Autodesk Inventor part; units mm, degrees
ref_plane "Work Plane1" through (-5, 47, 0) normal (0.7071, 0.7071, 0) x (0, 0, -1)
ref_plane "CentrePlane" through (8, 0, 0) normal (1, 0, 0) x (0, 0, -1)
ref_plane "YZ Plane" through (0, 0, 0) normal (1, 0, 0) x (0, 1, 0)
sketch "Sketch1" plane through (0, 0, 0) normal (0, 0, 1) x (1, 0, 0)
  line L0 (0, 0) -> (16, 0) construction
  line L1 (16, 0) -> (16, 8) construction
  line L2 (0, 8) -> (0, 0) construction
  line L3 (5.5, 10.5) -> (0, 10.5) construction
  line L4 (0, 10.5) -> (0, 8) construction
  line L5 (13.5, 10.5) -> (16, 10.5) construction
  line L6 (16, 10.5) -> (16, 8) construction
  line L7 (6.5, 37) -> (12.5, 37) construction
  line L8 (12.5, 37) -> (12.5, 8) construction
  line L9 (12.5, 8) -> (6.5, 8) construction
  line L10 (6.5, 8) -> (6.5, 37) construction
  line L11 (0.5, 34.5) -> (15.5, 34.5) construction
  line L12 (15.5, 34.5) -> (15.5, 10.5) construction
  line L13 (15.5, 10.5) -> (0.5, 10.5) construction
  line L14 (0.5, 10.5) -> (0.5, 34.5) construction
  line L15 (-2, 0) -> (-2, 39)
  line L16 (-2, 39) -> (18, 39)
  line L17 (8, -29.8106) -> (8, -55.1885) construction
  line L18 (-5, 47) -> (-5, 0)
  line L19 (-2, 0) -> (-5, 0)
  line L20 (-5, 47) -> (10, 47)
  line L21 (21, 47) -> (21, 0)
  line L22 (18, 0) -> (21, 0)
  line L23 (21, 47) -> (10, 47)
  line L24 (18, 0) -> (18, 39)
  line L25 (16.05, 25.6) -> (16.05, 19.4) construction
  line L26 (-0.05, 19.4) -> (-0.05, 25.6) construction
  line L27 (-0.05, 25.6) -> (0.5, 25.6) construction
  line L28 (16.05, 25.6) -> (15.5, 25.6) construction
  line L29 (16.05, 19.4) -> (15.5, 19.4) construction
  line L30 (-0.05, 19.4) -> (0.5, 19.4) construction
  line L31 (16.05, 22.5) -> (-0.05, 22.5) construction
  line L32 (0, 8) -> (16, 8) construction
  line L33 (5.5, 10.5) -> (5.5, 8) construction
  line L34 (13.5, 10.5) -> (13.5, 8) construction
  line L35 (5.5, 8) -> (13.5, 8) construction
  point P0 (6.5, 22.5)
  point P1 (0.5, 22.5)
  point P2 (9.5, 8)
  point P3 (8, 0)
  point P4 (8, 39)
  point P5 (8, -42.4996)
  point P6 (9.5, 8)
  point P7 (8, 22.5)
  dimension "d1" = 16
  dimension "d7" = 6
  dimension "d9" = 6
  dimension "d10" = 3
  dimension "d11" = 29
  dimension "d12" = 24
  dimension "d20" = 2
  dimension "thickness" = 3
  dimension "d23" = 8
  dimension "d31" = 22.5
  dimension "d40" = 24.5
  dimension "d41" = 39
  dimension "d60" = 6.2
  dimension "d62" = 16.1
  dimension "d63" = 8
  dimension "d64" = 8
  dimension "d65" = 1
  dimension "d66" = 2.5
  dimension "d97" = 2
extrude "LENGTH" add sketch "Sketch1" against normal blind 73.5
sketch "Sketch2" plane through (-5, 0, 0) normal (-1, 0, 0) x (0, 0, 1)
  circle A0 centre (-12, 22.5) radius 3
  circle A1 centre (-61.5, 22.5) radius 3
  line L0 (-73.5, 0) -> (-73.5, 47) construction
  line L1 (0, 47) -> (0, 0) construction
  dimension "d26" = 6
  dimension "d28" = 6
  dimension "d29" = 12
  dimension "d30" = 12
  dimension "d32" = 22.5
extrude "Extrusion2" cut sketch "Sketch2" against normal through all
ref_plane "Work Plane1" through (-5, 47, 0) normal (0.7071, 0.7071, 0) x (0, 0, -1)
ref_plane "CentrePlane" through (8, 0, 0) normal (1, 0, 0) x (0, 0, -1)
sketch "Measurements" plane through (-5, 0, 0) normal (-1, 0, 0) x (0, 0, 1)
  line L0 (-18.9044, 8) -> (-18.9044, 0) construction
  line L1 (0, 0) -> (0, 8) construction
  spline S0 degree 3 poles (-18.9044, 0) (-18.8729, 0.004) (-18.7747, 0.0145) (-18.6089, 0.0198) (-18.4076, 0.0173) (-18.2077, -0.0064) (-18.0095, -0.0413) (-17.7511, -0.1137) (-17.4304, -0.2111) (-17.1073, -0.2999) (-16.8501, -0.3765) (-16.6638, -0.4528) (-16.4821, -0.5394) (-16.3106, -0.6447) (-16.1439, -0.7575) (-15.9893, -0.8866) (-15.8435, -1.0251) (-15.7068, -1.1728) (-15.5834, -1.3319) (-15.4695, -1.4977) (-15.3662, -1.6705) (-15.2464, -1.9105) (-15.1208, -2.2219) (-15.0142, -2.6104) (-14.9462, -3.0072) (-14.9104, -3.408) (-14.9034, -3.8104) (-14.9258, -4.2123) (-14.9692, -4.6123) (-15.0344, -5.0094) (-15.0913, -5.2714) (-15.1198, -5.4024) knots -0.847201 -0.847201 -0.847201 -0.847201 -0.83705 -0.815587 -0.794126 -0.772659 -0.751201 -0.729734 -0.686802 -0.64387 -0.622403 -0.600945 -0.579478 -0.558017 -0.536554 -0.515088 -0.49363 -0.472163 -0.450698 -0.429238 -0.407769 -0.386302 -0.343394 -0.300476 -0.257562 -0.214646 -0.17172 -0.12879 -0.085861 -0.04293 0 0 0 0 construction
  spline S1 degree 3 poles (-4.5152, -5.4024) (-4.5336, -5.2605) (-4.5704, -4.9766) (-4.6037, -4.5484) (-4.6135, -4.119) (-4.6009, -3.6896) (-4.557, -3.2623) (-4.4825, -2.8392) (-4.3742, -2.4233) (-4.2256, -2.0199) (-4.0637, -1.7) (-3.9145, -1.4557) (-3.7891, -1.2813) (-3.6528, -1.1153) (-3.5072, -0.9573) (-3.3484, -0.8126) (-3.1807, -0.6785) (-3.0046, -0.5552) (-2.8172, -0.4504) (-2.6251, -0.3539) (-2.424, -0.2783) (-2.219, -0.214) (-1.9385, -0.1559) (-1.5868, -0.0908) (-1.2369, -0.0163) (-0.9555, 0.0373) (-0.7415, 0.0564) (-0.5268, 0.0635) (-0.3125, 0.0479) (-0.1366, 0.0272) (-0.0331, 0.0071) (0, 0) knots -1.373604 -1.373604 -1.373604 -1.373604 -1.330674 -1.287743 -1.244814 -1.201884 -1.158958 -1.116042 -1.073128 -1.03021 -0.987302 -0.965835 -0.944366 -0.922906 -0.901441 -0.879974 -0.858516 -0.83705 -0.815587 -0.794126 -0.772659 -0.751201 -0.729734 -0.686802 -0.64387 -0.622403 -0.600945 -0.579478 -0.558017 -0.536554 -0.526403 -0.526403 -0.526403 -0.526403 construction
  spline S2 degree 3 poles (-7.7374, -14.9236) (-7.6284, -14.7418) (-7.4104, -14.3783) (-7.0987, -13.824) (-6.7983, -13.2636) (-6.5111, -12.6963) (-6.2373, -12.1224) (-5.9778, -11.5419) (-5.7335, -10.9548) (-5.5053, -10.3613) (-5.2945, -9.7613) (-5.1024, -9.1551) (-4.9307, -8.5428) (-4.7815, -7.9246) (-4.6579, -7.3008) (-4.5633, -6.6718) (-4.516, -6.1439) (-4.4999, -5.72) (-4.5101, -5.5083) (-4.5152, -5.4024) knots -1.017256 -1.017256 -1.017256 -1.017256 -0.953675 -0.890094 -0.826513 -0.762932 -0.699351 -0.63577 -0.572189 -0.508609 -0.445029 -0.381449 -0.31787 -0.254291 -0.190714 -0.127139 -0.063568 -0.03178 0 0 0 0 construction
  arc A0 (-11.8976, -14.9236) -> (-7.7374, -14.9236) centre (-9.8175, 41.288) ccw construction
  spline S3 degree 3 poles (-15.1198, -5.4024) (-15.1249, -5.5083) (-15.1352, -5.72) (-15.119, -6.1439) (-15.0717, -6.6718) (-14.9771, -7.3008) (-14.8535, -7.9246) (-14.7043, -8.5428) (-14.5326, -9.1551) (-14.3405, -9.7613) (-14.1297, -10.3613) (-13.9015, -10.9548) (-13.6572, -11.5419) (-13.3977, -12.1224) (-13.1239, -12.6963) (-12.8366, -13.2636) (-12.5363, -13.824) (-12.2245, -14.3782) (-12.0065, -14.7418) (-11.8976, -14.9236) knots -1.017256 -1.017256 -1.017256 -1.017256 -0.985476 -0.953687 -0.890117 -0.826542 -0.762964 -0.699386 -0.635807 -0.572227 -0.508647 -0.445066 -0.381486 -0.317905 -0.254324 -0.190743 -0.127162 -0.063581 0 0 0 0 construction
  line L2 (-18.9044, 8) -> (0, 8) construction
  line L3 (0, 43) -> (0, 0) construction
  circle A1 centre (-9.8175, -59.712) radius 50 construction
  line L4 (0, 0) -> (-73.5, 0)
  circle A2 centre (-12, 22.5) radius 3
  circle A3 centre (-61.5, 22.5) radius 3
  circle A4 centre (-12, 22.5) radius 14.5
  circle A5 centre (-61.5, 22.5) radius 14.5
  point P0 (-9.8175, -14.962)
  dimension "d42" = 8
  dimension "d43" = 100
  dimension "d44" = 44.75
  dimension "d46" = 9.8175
  dimension "d47" = 14.962
  dimension "d49" = 59.712
  dimension "d67" = 29
  dimension "d68" = 29
sketch "Sketch5" plane through (-5, 0, 0) normal (-1, 0, 0) x (0, 0, 1)
  circle A0 centre (-36.75, -59.712) radius 50 construction
  line L0 (0, 0) -> (-73.5, 0)
  circle A1 centre (-36.75, -59.712) radius 5
  line L1 (-73.5, 0) -> (-48.8926, -64.355)
  arc A2 (-48.8926, -64.355) -> (-24.6074, -64.355) centre (-36.75, -59.712) ccw
  line L2 (-24.6074, -64.355) -> (0, 0)
  point P0 (-36.75, 0)
  dimension "d50" = 59.712
  dimension "d51" = 100
  dimension "bearingOD" = 10
  dimension "d53" = 8
extrude "Extrusion4" add sketch "Sketch5" against normal up to surface (3 mm away)
mirror "Mirror2" about plane through (8, 0, 0) normal (1, 0, 0) of "Extrusion4"
sketch "Sketch6" plane through (-2, 39, 0) normal (1, 0, 0) x (0, 0, -1)
  line L0 (0, 0) -> (73.5, 0)
  circle A0 centre (12, -16.5) radius 3
  circle A1 centre (12, -16.5) radius 3
  circle A2 centre (12, -16.5) radius 14.5
  circle A3 centre (61.5, -16.5) radius 14.5
  circle A4 centre (36.75, -98.712) radius 5
  circle A5 centre (12, -16.5) radius 3
  circle A6 centre (61.5, -16.5) radius 3
  line L1 (0, 8) -> (0, -39)
  line L2 (0, 8) -> (73.5, 8)
  line L3 (73.5, -39) -> (73.5, 8)
  line L4 (73.5, -39) -> (48.8926, -103.355)
  arc A7 (24.6074, -103.355) -> (48.8926, -103.355) centre (36.75, -98.712) ccw
  line L5 (24.6074, -103.355) -> (0, -39)
  line L6 (31.75, -22) -> (41.75, -22)
  arc A8 (46.75, 0) -> (41.75, -22) centre (92.65, -22) ccw
  line L7 (36.75, -22) -> (36.75, 0)
  arc A9 (31.75, -22) -> (26.75, 0) centre (-19.15, -22) ccw
  line L8 (41.75, -22) -> (41.75, -11.9859) construction
  line L9 (36.75, 0) -> (46.75, 0) construction
  line L10 (-19.15, 23.5572) -> (92.65, 23.5572)
  line L11 (92.65, 23.5572) -> (92.65, -126.6469)
  line L12 (92.65, -126.6469) -> (-19.15, -126.6469)
  line L13 (-19.15, -126.6469) -> (-19.15, 23.5572)
  point P0 (26.75, 0)
  dimension "d70" = 30
  dimension "d72" = 10
  dimension "d74" = 10
extrude "Extrusion5" add sketch "Sketch6" along normal up to surface (20 mm away) contours L0 L7 L6 A9 | L0 A8 L6 L7
extrude "Extrusion6" cut sketch "Sketch6" against normal blind 10 contours L1 L2 L3 L0 | L0 A9 L6 A8 L3 A3 L4 A7 L5 L1 A2 | L0 L7 L6 A9 | L1 A2 | A2 L1 | L0 A8 L6 L7 | L3 A3 | A3 L3 | A0 | A4 | A6 | L10 L11 L12 L13
mirror "Mirror3" about plane through (8, 0, 0) normal (1, 0, 0) of "Extrusion6"
sketch "Sketch8" plane through (18, 39, -73.5) normal (1, 0, 0) x (0, 0, -1)
  circle A0 centre (-67.5, 4) radius 3.36
  circle A1 centre (-36.75, -16) radius 3.36
  line L0 (-73.5, 8) -> (0, 8)
  line L1 (-73.5, 0) -> (-73.5, 8)
  line L2 (-41.75, -22) -> (-31.75, -22)
  line L3 (-36.75, 21.8835) -> (-36.75, 39.4907)
  circle A2 centre (-6, 4) radius 3.36
  point P0 (-73.5, -39)
  point P1 (-36.75, 8)
  point P2 (-73.5, 4)
  point P3 (-36.75, 8)
  dimension "d79" = 6.72
  dimension "d80" = 6
  dimension "d81" = 6
hole "Hole1" at (18, 43, -6) at (18, 43, -67.5) at (18, 23, -36.75) direction (-1, 0, 0) diameter 3 depth 7 tip angle 118
thread "Thread1"
thread "Thread2"
thread "Thread3"
mirror "Mirror4" about plane through (8, 0, 0) normal (1, 0, 0) of "Hole1"
fillet "Fillet3" radius 3 2 edges at (8, 39, -46.75) (8, 39, -26.75)
fillet "Fillet4" radius 3 4 edges at (8, 47, 0) (8, 47, -73.5) (8, 39, 0) (8, 39, -73.5)
equation "\"d23\" = d0"
equation "\"tol\" = 1"
properties part number "trolley6mm-centre"
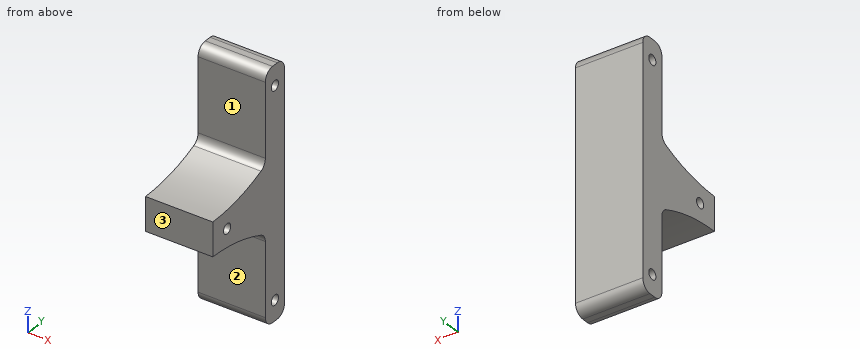
Work out the finished part from the listing and answer in its coordinate system (mm). Face numbers are marked on the shaded views. A direction names the side the tool comes from. Coordinates: 2 decimals unless noted, no trailing zeros. Loops run counter-clockwise (first coordinate to the right, second up) from the corner with the lowest first, then second, coordinate; pieces in that order, holes last.
1) Section A-A (x = 13.25) is taken. Give the vertices of the cut face in (y, z).
Results:
outline: (17, -41.75) arc R50.9 cw to (37.19, -45.93) arc R3 cw to (39, -48.68) - (39, -70.5) arc R3 ccw to (42, -73.5) - (44, -73.5) arc R3 ccw to (47, -70.5) - (47, -3) arc R3 ccw to (44, 0) - (42, 0) arc R3 ccw to (39, -3) - (39, -24.82) arc R3 cw to (37.19, -27.57) arc R50.9 cw to (17, -31.75) - close; hole circle Ø3 at (23, -36.75); hole circle Ø3 at (43, -67.5); hole circle Ø3 at (43, -6)
2) Section C-C (y = 34.5) is taken. Give the vertices of the cut face in (x, z), plus the area to 3 significant figures.
Results:
outline: (-2, -44.85) - (18, -44.85) - (18, -28.65) - (-2, -28.65) - close
area: 324 mm2
3) Flat-ended cylindrical pins translate along their axes: pin 1 (1 mm diameter, centred on x = 8.5, z = -16, fed in from -Y); pin 2 (2.5 mm diameter, centred on y = 23, z = -36.75, fed in from +X); pin 3 (1.8 mm diameter, centred on y = 43, z = -6, fed in from -X). Find the tip coordinate at first contact, or state that the pin passes through.
Results:
pin 1: stops at y = 39
pin 2: stops at x = 10.85
pin 3: stops at x = 5.36
4) Section B-B (z = -52) is taken. Give the vertices of the cut face in (x, y).
Results:
outline: (-2, 39) - (18, 39) - (18, 47) - (-2, 47) - close
5) Consider probe 1 along Z at (x, y) = (2.5, 43); probe 2 along Y at (x, z) = (1.5, -6); probe 3 along Y at (x, z) = (14.75, -36.75). Determine where each line is inside the solid, lowest interval first.
Results:
probe 1: z = -73.5 to -69, -66 to -7.5, -4.5 to 0
probe 2: y = 39 to 41.5, 44.5 to 47
probe 3: y = 17 to 21.5, 24.5 to 47
6) For the marked faces 1, 2 and 3, determine the directions among +Z, -Z, +X, -X, +Y, -Y from which every point of the face is accessible in a straight line to the end or side of a thin tool.
Results:
face 1: +Z, +X, -X, -Y
face 2: -Z, +X, -X, -Y
face 3: +Z, -Z, +X, -X, -Y
